```python
from build123d import *

# Parameters (mm, degrees)
SKETCH2_R          = 2
SKETCH3_R          = 2
CUT_EXTRUDE1_DEPTH = 51


with BuildPart() as part:
    # Sketch1 → Revolve1 (revolve)
    with BuildSketch(Plane(origin=(0, 0, 0), x_dir=(0, 0, -1), z_dir=(1, 0, 0))):
        with BuildLine():
            Line((0, 0), (0, 50))
            ThreePointArc((0, 50), (5.523447707, 49.745221779), (10.999986942, 48.983050847))
            ThreePointArc((10.999986942, 48.983050847), (11.700701157, 48.467397387), (11.732280918, 47.597971357))
            ThreePointArc((11.732280918, 47.597971357), (8.591312849, 27.196972532), (16.039707174, 7.946313959))
            ThreePointArc((16.039707174, 7.946313959), (16.457104991, 2.734119354), (12, 0))
            Line((12, 0), (0, 0))
        make_face()
    revolve(axis=Axis((0, 0, 0), (0, 1, 0)))

    # Sketch2 → Cut-Revolve1 (revolve, cut)
    with BuildSketch(Plane(origin=(0, 0, 0), x_dir=(0, 0, -1), z_dir=(1, 0, 0))):
        with Locations((14.901947009, 9.591154926)):
            Circle(SKETCH2_R)
    revolve(axis=Axis((0, 0, 0), (0, 1, 0)), mode=Mode.SUBTRACT)

    # Sketch3 → Cut-Extrude1 (cut, through all)
    with BuildSketch(Plane.XZ):
        Circle(SKETCH3_R)
    extrude(amount=-CUT_EXTRUDE1_DEPTH, mode=Mode.SUBTRACT)


solid = part.part
```
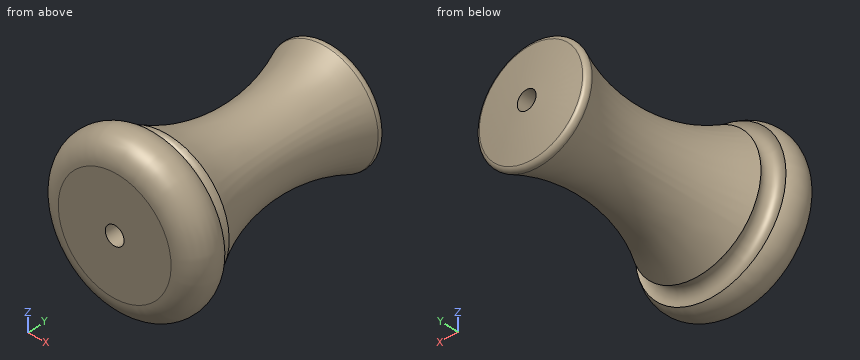
Design review of the part built by this model. Coordinates are the model's own, in mm. Give positions to 0.01 mm unless a question says otherwise; leave off trailing zeros. Order: outer loops, then holes, each group sorted by start corner. A loop starts at its lowest first (then second) coordinate and runs counter-clockwise, first axis right, second up. Notation, with made-up numbers: M -23.75,-24 L 19.25,-24 A17 ccw 19.25,-14 Z; hole C 55.5,-11 d2. An arc over 180 degrees is marked long. One line per question, with ' | ' between items. Start each with the question number.
Q1. We need section B-B (z = 0). Write out the cut boundary in (x, y).
Q2. We need section A-A (x = 0). Write out the cut boundary in (y, z), plus the area to 3 significant figures.
Q3. For L1, parallel to X at y = 16, z = 0; L2, parallel to Z at x = 0, y = 7; L3, parallel to Z at x = 0, y = 27, list the stretches that pass through material, from the lowest coordinate up. Write a range as [from, to].
Q4. We need section C-C (y = 14). Write out the cut boundary in (x, z).
Q5. We need section D-D (y = 41). Write out the cut boundary in (x, z), plus the area to 3 significant figures.
Q6. For pin 1 Ø8 at (x, z) = (-7.5, 2) entering from +Y; pin 2 Ø3 at (x, y) = (-7.5, 44.5) entering from -Z; pin 3 Ø3 at (x, y) = (10, 7) entering from -Z, all flat-tipped, find the tip position at first contact; note any pin that passes through.
Returned:
1) outline: M -16.04,7.95 A5 ccw -12,0 L -2,0 L -2,49.97 A60 ccw -11,48.98 A1 ccw -11.73,47.6 A40 cw -13.85,11.29 A2 cw long Z; M 2,0 L 12,0 A5 ccw 16.04,7.95 A2 cw long 13.85,11.29 A40 cw 11.73,47.6 A1 ccw 11,48.98 A60 ccw 2,49.97 Z
2) outline: M 0,-12 A5 ccw 7.95,-16.04 A2 cw long 11.29,-13.85 A40 cw 47.6,-11.73 A1 ccw 48.98,-11 A60 ccw 49.97,-2 L 0,-2 Z; M 0,2 L 49.97,2 A60 ccw 48.98,11 A1 ccw 47.6,11.73 A40 cw 11.29,13.85 A2 cw long 7.95,16.04 A5 ccw 0,12 Z | area: 906 mm2
3) L1: [-11.49, -2], [2, 11.49] | L2: [-16.58, -2], [2, 16.58] | L3: [-8.61, -2], [2, 8.61]
4) outline: C 0,0 d24.79; hole C 0,0 d4
5) outline: C 0,0 d19; hole C 0,0 d4 | area: 271 mm2
6) pin 1: y = 49.88 | pin 2: z = -8.83 | pin 3: z = -14.42
